from build123d import *

# Parameters (mm, degrees)
CUT_EXTRUDE1_DEPTH      = 21.305178915
CUT_EXTRUDE1_DEPTH_BACK = 21.305178915
SKETCH2_W               = 2
SKETCH2_H               = 1


with BuildPart() as part:
    # Sketch1 → Revolve1 (revolve)
    with BuildSketch(Plane.XY):
        Polygon((-6.5, 0), (-3.3, -3.2), (-3.3, -16.2), (0, -18.105255888), (0, 0), align=None)
    revolve(axis=Axis((0, 0, 0), (0, -1, 0)))

    # Sketch2 → Cut-Extrude1 (cut, two sides: drawn at the far end of the back side and taken through both)
    with BuildSketch(Plane.XY.offset(-CUT_EXTRUDE1_DEPTH_BACK)):
        with Locations((0, -0.5)):
            Rectangle(SKETCH2_W, SKETCH2_H)
    extrude(amount=CUT_EXTRUDE1_DEPTH + CUT_EXTRUDE1_DEPTH_BACK, mode=Mode.SUBTRACT)


solid = part.part
Work out the finished part from the listing and answer in its coordinate system (mm). A direction names the side the tool comes from. Give positions to 0.01 mm unless a question says otherwise; leave off trailing zeros. Order: outer loops, then holes, each group sorted by start corner. A loop starts at its lowest first (then second) coordinate and runs counter-clockwise, first axis right, second up. Notation, with made-up numbers: (18.5, 35.5) -> (53.5, 35.5) arc R35 cw to (53.5, 71.5) -> close; hole circle Ø5 at (-18.75, 36.5). An arc over 180 degrees is marked (long way). Answer as a JSON object with one key per item and string values. Group by question number.
1. The mould has two halves that part along X. Classify faces 1 (the conical face through (-0.5, -17.8, -0.16)), 2 (the flat face through (3, 0, 0)), 3 (the flat face through (-1, -0.5, -0.1)): released by +X, released by -X, zero draft, split by the parting line, or undercut.
2. A tool of negligible diameter and unlimited length cuts with its end or side. For faces 4 (the cylindrical face through (2.43, -9.79, -2.23)), 5 (the flat face through (-3, 0, 0)), 6 (the flat face through (0, -1, 0)), from which of +Z, -Z, +X, -X, +Y, -Y can it reach the whole face along a straight path? Write none if from no direction.
3. Section A-A on y = -15.75 is taken. Determine the outline of the cut face in (x, z).
4. Consider line 1 along X through (y, z) = (-10.5, 0); line 2 along Y through (x, z) = (3.25, -1). Determine where each line is inside the solid, lowest interval first. Write a range as [from, to].
5. Flat-ended cylindrical pins translate along their axes: pin 1 Ø0.8 at (y, z) = (-0.5, 3) entering from +X; pin 2 Ø5 at (x, z) = (0.5, -3.5) entering from -Y; pin 3 Ø1 at (x, y) = (1, -8.5) entering from -Z. Find the tip coordinate at first contact, or state that the pin passes through.
Result sheet:
{
 "1": {"face 1": "split by the parting line", "face 2": "zero draft", "face 3": "undercut"},
 "2": {"face 4": "-Y", "face 5": "+Z, -Z, +X, -X, +Y", "face 6": "+Z, -Z, +Y"},
 "3": {"outline": "circle Ø6.6 at (0, 0)"},
 "4": {"line 1": "x = [-3.3, 3.3]", "line 2": "y = [-3.1, 0]"},
 "5": {"pin 1": "stops at x = 5.7", "pin 2": "stops at y = -17.51", "pin 3": "stops at z = -3.26"}
}
